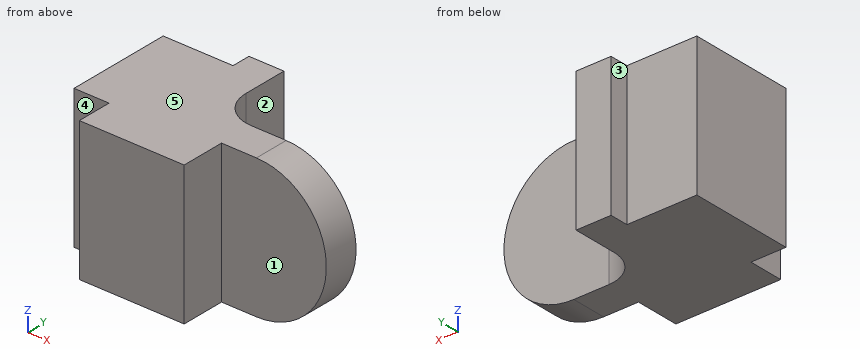
from build123d import *

# Parameters (mm, degrees)
BOSS_EXTRUDE1_DEPTH = 40
SKETCH3_OUTSIDE_W   = 90.5
SKETCH3_OUTSIDE_H   = 60.5
CUT_EXTRUDE1_DEPTH  = 40


with BuildPart() as part:
    # Sketch1 → Boss-Extrude1 (new body)
    with BuildSketch(Plane.XY):
        with BuildLine():
            Line((-15.809128631, 23.900414938), (-5.809128631, 23.900414938))
            Line((-5.809128631, 23.900414938), (-5.809128631, 11.12033195))
            ThreePointArc((-5.809128631, 11.12033195), (-2.880196443, 4.049264138), (4.190871369, 1.12033195))
            Line((4.190871369, 1.12033195), (34.190871369, 1.12033195))
            Line((34.190871369, 1.12033195), (34.190871369, -8.87966805))
            Line((34.190871369, -8.87966805), (4.190871369, -8.87966805))
            Line((4.190871369, -8.87966805), (4.190871369, -21.452282158))
            Line((4.190871369, -21.452282158), (-25.809128631, -21.452282158))
            Line((-25.809128631, -21.452282158), (-25.809128631, -11.452282158))
            Line((-25.809128631, -11.452282158), (-35.809128631, -11.452282158))
            Line((-35.809128631, -11.452282158), (-35.809128631, 18.547717842))
            Line((-35.809128631, 18.547717842), (-15.809128631, 18.547717842))
            Line((-15.809128631, 18.547717842), (-15.809128631, 23.900414938))
        make_face()
    extrude(amount=BOSS_EXTRUDE1_DEPTH)

    # Sketch3 outside → Cut-Extrude1 (cut)
    with BuildSketch(Plane(origin=(0, 1.12033195, 0), x_dir=(1, 0, 0), z_dir=(0, 1, 0))):
        with Locations((-0.809, -20)):
            Rectangle(SKETCH3_OUTSIDE_W, SKETCH3_OUTSIDE_H)
        with BuildLine():
            Line((14.190871369, 0), (-35.809128631, 0))
            Line((-35.809128631, 0), (-35.809128631, -40))
            Line((-35.809128631, -40), (14.190871369, -40))
            ThreePointArc((14.190871369, -40), (34.190871369, -20), (14.190871369, 0))
        make_face(mode=Mode.SUBTRACT)
    extrude(amount=-CUT_EXTRUDE1_DEPTH, mode=Mode.SUBTRACT)


solid = part.part
Verification items for the finished model (mm, model axes). Face numbers are marked on the shaded views. A direction names the side the tool comes from. Coordinates: 2 decimals unless noted, no trailing zeros. Order: outer loops, then holes, each group sorted by start corner. A loop starts at its lowest first (then second) coordinate and runs counter-clockwise, first axis right, second up. Notation, with made-up numbers: M 51.5,-5 L 83.5,-5 A25 ccw 83.5,21 Z; hole C -9.5,-31 d6. An arc over 180 degrees is marked long. One line per item, written item: value. Start each with the question number.
Item 1: Sectioned sample at A-A (z = 20). Enter the section's corners in (x, y), then the cut area to 3 significant figures.
Item 2: Sectioned sample at C-C (y = -5). Enter the section's corners in (x, z), then the cut area to 3 significant figures.
Item 3: Gauge pin test, flat ends, axial feed: pin 1 (3 mm diameter, centred on x = -29.5, z = 27, fed in from -Y); pin 2 (8 mm diameter, centred on x = -18.5, z = 22.5, fed in from +Y); pin 3 (6 mm diameter, centred on y = -16, z = 26.5, fed in from +X); pin 4 (6 mm diameter, centred on y = 22, z = 23.5, fed in from -X). Record the tip position at first contact, or that the pin passes through.
Item 4: Sectioned sample at B-B (x = -20). Enter the section's corners in (y, z), then the cut area to 3 significant figures.
Item 5: Sectioned sample at D-D (z = 32.5). Enter the section's corners in (x, y).
Item 6: Scan lines: probe 1 along Y at (x, z) = (8, 33); probe 2 along X at (y, z) = (16.5, 35); probe 3 along Y at (x, z) = (-26.5, 11.5). Record each from-to range of solid material in increasing order.
Item 7: Access from +Z, -Z, +X, -X, +Y, -Y to the whole of each face (thin tool, end or side, straight path). Record for the marked faces 1, 2, 3, 4 and 5.
Conclusion:
1. outline: M -35.81,-11.45 L -25.81,-11.45 L -25.81,-21.45 L 4.19,-21.45 L 4.19,-8.88 L 34.19,-8.88 L 34.19,1.12 L 4.19,1.12 A10 cw -5.81,11.12 L -5.81,23.9 L -15.81,23.9 L -15.81,18.55 L -35.81,18.55 Z
1. area: 1,700 mm^2
2. outline: M -35.81,0 L 14.19,0 A20 ccw 14.19,40 L -35.81,40 Z
2. area: 2,630 mm^2
3. pin 1: stops at y = -11.45
3. pin 2: stops at y = 23.9
3. pin 3: stops at x = 4.19
3. pin 4: stops at x = -15.81
4. outline: M -21.45,0 L 18.55,0 L 18.55,40 L -21.45,40 Z
4. area: 1,600 mm^2
5. outline: M -35.81,-11.45 L -25.81,-11.45 L -25.81,-21.45 L 4.19,-21.45 L 4.19,-8.88 L 29.8,-8.88 L 29.8,1.12 L 4.19,1.12 A10 cw -5.81,11.12 L -5.81,23.9 L -15.81,23.9 L -15.81,18.55 L -35.81,18.55 Z
6. probe 1: y = -8.88 to 1.12
6. probe 2: x = -35.81 to -5.81
6. probe 3: y = -11.45 to 18.55
7. face 1: +Z, -Z, +X, -Y
7. face 2: +Z, -Z, +X, +Y
7. face 3: +Z, -Z, -X, +Y
7. face 4: +Z, -Z, -X, -Y
7. face 5: +Z, +X, -X, +Y, -Y
